from build123d import *

# Parameters (mm, degrees)
SKETCH1_W                    = 80
SKETCH1_H                    = 38
BOSS_EXTRUDE1_DEPTH          = 3
M1_6X0_35_TAPPED_HOLE1_D     = 1.25
M1_6X0_35_TAPPED_HOLE1_DEPTH = 4.95
M1_6X0_35_TAPPED_HOLE1_TIP   = 0.375537887
FILLET1_R                    = 3
SKETCH6_W                    = 19.2
SKETCH6_H                    = 8.035
CUT_EXTRUDE1_DEPTH           = 45.384682042
FILLET2_R                    = 0.5
LPATTERN1_COUNT              = 2
LPATTERN1_PITCH              = 47.267
FILLET2_OF_LPATTERN1_R       = 0.5
MIRROR1_DEPTH                = 3
M1_6_CLEARANCE_HOLE3_D       = 1.8
M1_6_CLEARANCE_HOLE3_DEPTH   = 4.25
M1_6_CLEARANCE_HOLE3_TIP     = 0.540774557
M2_5X0_45_TAPPED_HOLE1_D     = 2.05
M2_5X0_45_TAPPED_HOLE1_DEPTH = 7.25
M2_5X0_45_TAPPED_HOLE1_TIP   = 0.615882135
CUT_EXTRUDE2_DEPTH           = 45.384682042
CUT_EXTRUDE2_DEPTH_BACK      = 45.384682042
SKETCH16_R                   = 4
CHAMFER1_SIZE                = 0.5


# Read off the part's stored shape, not the designer's step: Mirror1
with BuildPart() as part:
    # Sketch1 → Boss-Extrude1 (new body)
    with BuildSketch(Plane(origin=(0, 0, 0), x_dir=(1, 0, 0), z_dir=(0, 1, 0))):
        Rectangle(SKETCH1_W, SKETCH1_H)
    extrude(amount=BOSS_EXTRUDE1_DEPTH)

    # M1.6x0.35 Tapped Hole1
    with Locations(Plane(origin=(0, 3, 0), x_dir=(1, 0, 0), z_dir=(0, 1, 0))):
        with Locations((-35, 15), (-12.267, 15), (-12.267, -15), (-35, -15), (12.267, -15), (35, -15), (35, 15), (12.267, 15)):
            Hole(M1_6X0_35_TAPPED_HOLE1_D / 2, depth=M1_6X0_35_TAPPED_HOLE1_DEPTH)
            with Locations((0, 0, -(M1_6X0_35_TAPPED_HOLE1_DEPTH + M1_6X0_35_TAPPED_HOLE1_TIP / 2))):  # 118° drill point
                Cone(0, M1_6X0_35_TAPPED_HOLE1_D / 2, M1_6X0_35_TAPPED_HOLE1_TIP, mode=Mode.SUBTRACT)

    # Fillet1
    fillet1_edges = [part.edges().sort_by_distance(p)[0] for p in [
        (40, 1.5, 19),
        (-40, 1.5, 19),
        (-40, 1.5, -19),
        (40, 1.5, -19),
    ]]
    fillet(fillet1_edges, radius=FILLET1_R)

    # Sketch6 → Cut-Extrude1 (cut, symmetric)
    with BuildSketch(Plane.XZ):
        with Locations((-23.657734471, -15)):
            Rectangle(SKETCH6_W, SKETCH6_H)
    cut_extrude1 = extrude(amount=CUT_EXTRUDE1_DEPTH, both=True, mode=Mode.SUBTRACT)

    # Fillet2
    fillet2_edges = [part.edges().sort_by_distance(p)[0] for p in [
        (-33.257734471, 1.5, -19),
        (-14.057734471, 1.5, -10.9825),
        (-33.257734471, 1.5, -10.9825),
        (-14.057734471, 1.5, -19),
    ]]
    fillet(fillet2_edges, radius=FILLET2_R)

    # LPattern1: Cut-Extrude1 ×2
    with Locations(*[(i * LPATTERN1_PITCH, 0, 0) for i in range(1, LPATTERN1_COUNT)]):
        add(cut_extrude1, mode=Mode.SUBTRACT)

    # Fillet2 of LPattern1
    fillet2_of_lpattern1_edges = [part.edges().sort_by_distance(p)[0] for p in [
        (14.009265529, 1.5, -19),
        (33.209265529, 1.5, -10.9825),
        (14.009265529, 1.5, -10.9825),
        (33.209265529, 1.5, -19),
    ]]
    fillet(fillet2_of_lpattern1_edges, radius=FILLET2_OF_LPATTERN1_R)

    # Mirror1 outline → Mirror1 (cut)
    with BuildSketch(Plane(origin=(0, 0, 0), x_dir=(1, 0, 0), z_dir=(0, 1, 0))):
        with BuildLine():
            ThreePointArc((-32.757734471, -10.9825), (-33.111287862, -11.128946609), (-33.257734471, -11.4825))
            Line((-33.257734471, -11.4825), (-33.257734471, -18.5))
            ThreePointArc((-33.257734471, -18.5), (-33.40418108, -18.853553391), (-33.757734471, -19))
            Line((-33.757734471, -19), (-13.557734471, -19))
            ThreePointArc((-13.557734471, -19), (-13.911287861, -18.853553391), (-14.057734471, -18.5))
            Line((-14.057734471, -18.5), (-14.057734471, -11.4825))
            ThreePointArc((-14.057734471, -11.4825), (-14.20418108, -11.128946609), (-14.557734471, -10.9825))
            Line((-14.557734471, -10.9825), (-32.757734471, -10.9825))
        make_face()
        with BuildLine():
            ThreePointArc((14.009265529, -18.5), (13.86281892, -18.853553391), (13.509265529, -19))
            Line((13.509265529, -19), (33.709265529, -19))
            ThreePointArc((33.709265529, -19), (33.355712139, -18.853553391), (33.209265529, -18.5))
            Line((33.209265529, -18.5), (33.209265529, -11.4825))
            ThreePointArc((33.209265529, -11.4825), (33.06281892, -11.128946609), (32.709265529, -10.9825))
            Line((32.709265529, -10.9825), (14.509265529, -10.9825))
            ThreePointArc((14.509265529, -10.9825), (14.155712139, -11.128946609), (14.009265529, -11.4825))
            Line((14.009265529, -11.4825), (14.009265529, -18.5))
        make_face()
    extrude(amount=MIRROR1_DEPTH, mode=Mode.SUBTRACT)

    # M1.6 Clearance Hole3
    with Locations(Plane(origin=(0, 3, 0), x_dir=(1, 0, 0), z_dir=(0, 1, 0))):
        with Locations((-38.5, 0), (0, 17.5), (38.5, 0), (0, -17.5)):
            Hole(M1_6_CLEARANCE_HOLE3_D / 2, depth=M1_6_CLEARANCE_HOLE3_DEPTH)
            with Locations((0, 0, -(M1_6_CLEARANCE_HOLE3_DEPTH + M1_6_CLEARANCE_HOLE3_TIP / 2))):  # 118° drill point
                Cone(0, M1_6_CLEARANCE_HOLE3_D / 2, M1_6_CLEARANCE_HOLE3_TIP, mode=Mode.SUBTRACT)

    # M2.5x0.45 Tapped Hole1
    with Locations(Plane(origin=(0, 3, 0), x_dir=(1, 0, 0), z_dir=(0, 1, 0))):
        with Locations((32, 8), (32, -8), (-32, 0)):
            Hole(M2_5X0_45_TAPPED_HOLE1_D / 2, depth=M2_5X0_45_TAPPED_HOLE1_DEPTH)
            with Locations((0, 0, -(M2_5X0_45_TAPPED_HOLE1_DEPTH + M2_5X0_45_TAPPED_HOLE1_TIP / 2))):  # 118° drill point
                Cone(0, M2_5X0_45_TAPPED_HOLE1_D / 2, M2_5X0_45_TAPPED_HOLE1_TIP, mode=Mode.SUBTRACT)

    # Sketch16 → Cut-Extrude2 (cut, two sides: drawn at the far end of the back side and taken through both)
    with BuildSketch(Plane(origin=(0, 3, 0), x_dir=(1, 0, 0), z_dir=(0, 1, 0)).offset(-CUT_EXTRUDE2_DEPTH_BACK)):
        with Locations(Location((18.5, 0, 0), (0, 0, 270))):
            Circle(SKETCH16_R)
    extrude(amount=CUT_EXTRUDE2_DEPTH + CUT_EXTRUDE2_DEPTH_BACK, mode=Mode.SUBTRACT)

    # Chamfer1
    chamfer1_edges = [part.edges().sort_by_distance(p)[0] for p in [
        (18.5, 0, -4),
        (18.5, 3, -4),
    ]]
    chamfer(chamfer1_edges, length=CHAMFER1_SIZE)


solid = part.part
For this review, take the finished solid that the model builds, in its own axes (mm). A direction names the side the tool comes from. Coordinates: 2 decimals unless noted, no trailing zeros. Order: outer loops, then holes, each group sorted by start corner. A loop starts at its lowest first (then second) coordinate and runs counter-clockwise, first axis right, second up. Notation, with made-up numbers: (-23.5, 38.25) - (-4.5, 38.25) arc R28 ccw to (-4.5, 73.25) - close; hole circle Ø6 at (44, 37.5). An arc over 180 degrees is marked (long way). Answer as CSV lines item,"result". Start each with the question number.
1) Machinability: for faces 4 (the flat face through (23, 1, -10.982)), 5 (the cylindrical face through (33.024, 1.479, -8.045)), 6 (the flat face through (24, 1, 10.982)), which of the approach directions +Z, -Z, +X, -X, +Y, -Y give a long, thin tool a straight path to every point of the face, cutting with its end or side? Answer none if there is none.
2) To check wall thickness, follow line 1 along X through (y, z) = (1.85, -13); line 2 along Z through (x, y) = (18.5, 1); line 3 along Z through (x, y) = (0, 2.05). State the ranges of each line that lie inside material, in increasing order. Write a range as [from, to].
3) Add section A-A (z = 0). State the section outline as (x, y) points (3 decimals).
4) Add section C-C (x = 18.5). State the section outline as (y, z) points.
5) Insertion check: P1, Ø1.6, axis at x = 35, z = 15, coming from the +Y side; P2, Ø1.5, axis at x = -26.5, y = 2, coming from the -Z side. Each pin has a flat end and moves straight along its axis. Give the tip position at first contact, or say it passes through.
6) Add section B-B (x = 0). State the section outline as (y, z) points.
7) Add section D-D (x = -38.5). State the section outline as (y, z) points, then the cut area to 3 significant figures.
8) Draft analysis for pull direction X (two halves, no side actions). For faces 1 (the flat face through (40, 1, 0)), 2 (the cylindrical face through (-30.976, 1.479, -0.045)), 3 (the flat face through (-1, 3, 0)), state which applies: +X half, -X half, draft (parallel to the pull), parting line (faces both ways), or undercut.
Result:
1,face 4,"-Z, +Y, -Y"
1,face 5,"+Y, -Y"
1,face 6,"+Z, +Y, -Y"
2,line 1,"[-40, -33.26], [-14.06, 14.01], [33.21, 40]"
2,line 2,"[-10.98, -4], [4, 10.98]"
2,line 3,"[-19, -18.4], [-16.6, 16.6], [18.4, 19]"
3,outline,"(-40, 0) - (-39.4, 0) - (-39.4, 3) - (-40, 3) - close; (-37.6, 0) - (-33.025, 0) - (-33.025, 3) - (-37.6, 3) - close; (-30.975, 0) - (14, 0) - (14.5, 0.5) - (14.5, 2.5) - (14, 3) - (-30.975, 3) - close; (22.5, 0.5) - (23, 0) - (37.6, 0) - (37.6, 3) - (23, 3) - (22.5, 2.5) - close; (39.4, 0) - (40, 0) - (40, 3) - (39.4, 3) - close"
4,outline,"(0, -10.98) - (3, -10.98) - (3, -4.5) - (2.5, -4) - (0.5, -4) - (0, -4.5) - close; (0, 4.5) - (0.5, 4) - (2.5, 4) - (3, 4.5) - (3, 10.98) - (0, 10.98) - close"
5,P1,"y = 3"
5,P2,"z = -10.98"
6,outline,"(0, -19) - (3, -19) - (3, -18.4) - (0, -18.4) - close; (0, -16.6) - (3, -16.6) - (3, 16.6) - (0, 16.6) - close; (0, 18.4) - (3, 18.4) - (3, 19) - (0, 19) - close"
7,outline,"(0, -18.6) - (3, -18.6) - (3, -0.9) - (0, -0.9) - close; (0, 0.9) - (3, 0.9) - (3, 18.6) - (0, 18.6) - close"
7,area,"106 mm^2"
8,face 1,"+X half"
8,face 2,"undercut"
8,face 3,"draft"
